Can you work these out from the model? Positions are in its coordinate system, mm. A direction names the side the tool comes from. Give positions to 0.01 mm unless a question says otherwise; leave off trailing zeros. Write each loop counter-clockwise with the first axis right and the second up, starting at its lowest first coordinate (ties: lowest second). Pieces come first, ordered by that corner, then holes.
1. Suppose I cut it at B-B (y = 10.5). Please give me the cut outline in (x, z), and give its area (3 significant figures).
2. I'm going to push a flat-ended pin straight in: pin 1 (3.5 mm diameter, centred on x = 170.5, y = 8, fed in from -Z). Where does the tip first touch, or does it pass through?
3. If I drill on probe 1 along X at (y, z) = (13.9, 7.5); probe 2 along Y at (x, z) = (201.5, 6.75), over which ranges is the centre line in solid material (lowest first)?
4. Suppose I cut it at A-A (x = 82). Please give me the cut outline in (y, z), and give its area (3 significant figures).
5. On a 3-axis mill with a long thin cutter (end or side, diameter ignored), from which of +Z, -Z, +X, -X, +Y, -Y can I reach the whole of each face in a straight line? I mean faces 5 (the flat face through (132, 7, 1.5)), 6 (the flat face through (128, 15, 7)). Say none if no direction works.
6. Thinking about a two-plate mould opening in Z: for faces 1 (the flat face through (132, 7, 13.5)), 2 (the flat face through (128, 8, 0)), 3 (the flat face through (128, 8, 15)), 4 (the flat face through (128, 0, 7)), which applies, pulls with the +Z half, pulls with the -Z half, needs draft (parallel to the pull), parting line crosses it, or undercut?
```python
from build123d import *

# Parameters (mm, degrees)
SKETCH_2_W          = 260
SKETCH_2_H          = 15
EXTRUDE_1_DEPTH     = 15
SKETCH_3_R          = 1.5
CUT_EXTRUDE_1_DEPTH = 261.863949215
SKETCH_4_W          = 12
SKETCH_4_H          = 12
CUT_EXTRUDE_2_DEPTH = 261.863949215


with BuildPart() as part:
    # ｽｹｯﾁ2 → ﾎﾞｽ - 押し出し1 (new body)
    with BuildSketch(Plane.XY):
        with Locations((130, 7.5)):
            Rectangle(SKETCH_2_W, SKETCH_2_H)
    extrude(amount=EXTRUDE_1_DEPTH)

    # ｽｹｯﾁ3 → ｶｯﾄ - 押し出し1 (cut, through all)
    with BuildSketch(Plane(origin=(0, 15, 0), x_dir=(1, 0, 0), z_dir=(0, 1, 0))):
        with Locations(Location((7.5, -7.5, 0), (0, 0, 270))):
            Circle(SKETCH_3_R)
        with Locations(Location((252.5, -7.5, 0), (0, 0, 270))):
            Circle(SKETCH_3_R)
    extrude(amount=-CUT_EXTRUDE_1_DEPTH, mode=Mode.SUBTRACT)

    # ｽｹｯﾁ4 → ｶｯﾄ - 押し出し2 (cut, through all)
    with BuildSketch(Plane(origin=(260, 0, 0), x_dir=(0, 0, -1), z_dir=(1, 0, 0))):
        with Locations((-7.5, 7.5)):
            Rectangle(SKETCH_4_W, SKETCH_4_H)
    extrude(amount=-CUT_EXTRUDE_2_DEPTH, mode=Mode.SUBTRACT)


solid = part.part
```
Checks:
1. outline: (0, 0) - (260, 0) - (260, 1.5) - (0, 1.5) - close; (0, 13.5) - (260, 13.5) - (260, 15) - (0, 15) - close
1. area: 780 mm2
2. pin 1: stops at z = 0
3. probe 1: x = 0 to 6, 9 to 251, 254 to 260
3. probe 2: y = 0 to 1.5, 13.5 to 15
4. outline: (0, 0) - (15, 0) - (15, 15) - (0, 15) - close; hole (1.5, 1.5) - (13.5, 1.5) - (13.5, 13.5) - (1.5, 13.5) - close
4. area: 81.0 mm2
5. face 5: +X, -X
5. face 6: +Z, -Z, +X, -X, +Y
6. face 1: undercut
6. face 2: pulls with the -Z half
6. face 3: pulls with the +Z half
6. face 4: needs draft
